Input: part model. Units: mm. Frame: model coordinates. A direction names the side the tool comes from. Round coordinates to 2 decimals unless told otherwise and drop trailing zeros. Loops run counter-clockwise (first coordinate to the right, second up) from the corner with the lowest first, then second, coordinate; pieces in that order, holes last. Notation, with made-up numbers: (71.25, -4.5) -> (108.25, -4.5) arc R16 ccw to (108.25, 1.5) -> close; hole circle Ø6 at (81, 53). An arc over 180 degrees is marked (long way). Answer as a JSON object with one key per item and string values.
```python
from build123d import *

# Parameters (mm, degrees)
F0_R     = 18
F1_DEPTH = 24
F2_R     = 2.5
F2_R_2   = 5.5
F3_DEPTH = 25
F4_R     = 9
F5_DEPTH = 11
F6_SIZE  = 0.5


with BuildPart() as f1:
    # F0 (on Front) → F1 (new body)
    with BuildSketch(Plane.XZ):
        Polygon((-30, -22), (30, -22), (75, 26), (75, 50), (0, 50), (-75, 50), (-75, 26), align=None)
        Circle(F0_R, mode=Mode.SUBTRACT)
    extrude(amount=F1_DEPTH)

    # F2 (on face) → F3 (cut)
    with BuildSketch(Plane.XZ.offset(24)):
        with Locations((-23.5, 0)):
            Circle(F2_R)
        with Locations((-16.617009, -16.617009)):
            Circle(F2_R)
        with Locations((16.617009, -16.617009)):
            Circle(F2_R)
        with Locations((23.5, 0)):
            Circle(F2_R)
        with Locations((16.617009, 16.617009)):
            Circle(F2_R)
        with Locations((-16.617009, 16.617009)):
            Circle(F2_R)
        with Locations((-62.5, 38)):
            Circle(F2_R_2)
        with Locations((-35, 38)):
            Circle(F2_R_2)
        with Locations((35, 38)):
            Circle(F2_R_2)
        with Locations((62.5, 38)):
            Circle(F2_R_2)
        with Locations((0, 38)):
            Circle(F2_R_2)
    extrude(amount=-F3_DEPTH, mode=Mode.SUBTRACT)

    # F4 (on face) → F5 (cut)
    with BuildSketch(Plane.XZ.offset(24)):
        with Locations((-62.5, 38)):
            Circle(F4_R)
        with Locations((-35, 38)):
            Circle(F4_R)
        with Locations((62.5, 38)):
            Circle(F4_R)
        with Locations((35, 38)):
            Circle(F4_R)
        with Locations((0, 38)):
            Circle(F4_R)
    extrude(amount=-F5_DEPTH, mode=Mode.SUBTRACT)

    # F6
    f6_edges = [f1.edges().sort_by_distance(p)[0] for p in [
        (-71.5, -24, 38),
        (-44, -24, 38),
        (-19.117009, -24, 16.617009),
        (-26, -24, 0),
        (-19.117009, -24, -16.617009),
        (-18, -24, 0),
        (14.117009, -24, 16.617009),
        (26, -24, 38),
        (53.5, -24, 38),
        (21, -24, 0),
        (14.117009, -24, -16.617009),
        (-68, 0, 38),
        (-40.5, 0, 38),
        (-19.117009, 0, 16.617009),
        (-26, 0, 0),
        (-19.117009, 0, -16.617009),
        (-18, 0, 0),
        (14.117009, 0, -16.617009),
        (21, 0, 0),
        (14.117009, 0, 16.617009),
        (29.5, 0, 38),
        (57, 0, 38),
        (-9, -24, 38),
        (-5.5, 0, 38),
    ]]
    chamfer(f6_edges, length=F6_SIZE)


solid = f1.part
```
1) Draft query along Z for faces 3 (the face through (-67, -13, 34)), 4 (the face through (1, -12, 50)). Return one class per face: +Z half, -Z half, draft (parallel to the pull), parting line (faces both ways), or undercut.
Output:
{"face 3": "undercut", "face 4": "+Z half"}
2) Section B-B, the plane z = 0. Output: boundary loops of the cut face in (x, y) (3 decimals).
Output:
{"outline": "(-50.625, -24) -> (-26.5, -24) -> (-26, -23.5) -> (-26, -0.5) -> (-26.5, 0) -> (-50.625, 0) -> close; (-21, -23.5) -> (-20.5, -24) -> (-18.5, -24) -> (-18, -23.5) -> (-18, -0.5) -> (-18.5, 0) -> (-20.5, 0) -> (-21, -0.5) -> close; (18, -23.5) -> (18.5, -24) -> (20.5, -24) -> (21, -23.5) -> (21, -0.5) -> (20.5, 0) -> (18.5, 0) -> (18, -0.5) -> close; (26, -23.5) -> (26.5, -24) -> (50.625, -24) -> (50.625, 0) -> (26.5, 0) -> (26, -0.5) -> close"}
3) Section A-A, the plane x = 62.5. Output: boundary loops of the cut face in (y, z).
Output:
{"outline": "(-24, 12.67) -> (0, 12.67) -> (0, 32) -> (-0.5, 32.5) -> (-13, 32.5) -> (-13, 29) -> (-23.5, 29) -> (-24, 28.5) -> close; (-24, 47.5) -> (-23.5, 47) -> (-13, 47) -> (-13, 43.5) -> (-0.5, 43.5) -> (0, 44) -> (0, 50) -> (-24, 50) -> close"}
4) Section C-C, the plane y = -9. Count the separate pieces of the cut face and the enclosed holes in it, plus the area to 3 significant figures.
Output:
{"separate pieces": "1", "enclosed holes": "12", "area": "7,030 mm^2"}
5) Ray query, probe 1 along Z at (x, y) = (23.5, -7); probe 2 along X at (y, z) = (-7.25, 43); probe 3 along X at (y, z) = (-13.5, 14.5). Return the intervals inside material, ascending.
Output:
{"probe 1": "z = -22 to -2.5, 2.5 to 50", "probe 2": "x = -75 to -64.79, -60.21 to -37.29, -32.71 to -2.29, 2.29 to 32.71, 37.29 to 60.21, 64.79 to 75", "probe 3": "x = -64.22 to -17.95, -15.29 to -10.67, 10.67 to 15.29, 17.95 to 64.22"}
6) Reachability of faces 1 (the face through (39, -13, 42)), 2 (the face through (-2.343, -11.839, 17.847)) from +Z, -Z, +X, -X, +Y, -Y: full face, straight path, thin tool, end or side. Return the list, or none.
Output:
{"face 1": "-Y", "face 2": "+Y, -Y"}
7) Section D-D, the plane x = -46.5. Output: boundary loops of the cut face in (y, z).
Output:
{"outline": "(-24, -4.4) -> (0, -4.4) -> (0, 50) -> (-24, 50) -> close"}
8) Contact query for flat-ended pins moving along their axis: P1, Ø17.5, axis at x = 0, z = 38, coming from the +Y side; P2, Ø12, axis at y = -5.5, z = -6.5, coming from the -X side; P3, Ø2, axis at y = -5.5, z = 22.5, coming from the -X side; P4, Ø1.5, axis at x = -45.5, y = -15.5, coming from the -Z side. Output: stop coordinate, or through.
Output:
{"P1": "stops at y = 0", "P2": "stops at x = -50.16", "P3": "stops at x = -72.66", "P4": "stops at z = -6.27"}
